Could you check a few things on this model? Use its own coordinates, in mm. A direction names the side the tool comes from. Give positions to 0.01 mm unless a question says otherwise; leave off trailing zeros. Loops run counter-clockwise (first coordinate to the right, second up) from the corner with the lowest first, then second, coordinate; pieces in that order, holes last. Notation, with made-up numbers: (56, -7.75) - (89, -7.75) arc R31 ccw to (89, 24.25) - close; hole circle Ø4 at (31, 22). An arc over 180 degrees is marked (long way). Use CSV: the item, a comma, the result in double quotes.
from build123d import *

# Parameters (mm, degrees)
SKETCH1_W           = 144
SKETCH1_H           = 125.68
BOSS_EXTRUDE1_DEPTH = 3
SKETCH2_W           = 144
SKETCH2_H           = 125.68
SKETCH2_W_2         = 140.282516161
SKETCH2_H_2         = 121.548177757
BOSS_EXTRUDE2_DEPTH = 83
SKETCH4_W           = 103.746737409
SKETCH4_H           = 37.953937335
CUT_EXTRUDE1_DEPTH  = 20
SKETCH5_W           = 110.713821745
SKETCH5_H           = 19.414835186
SKETCH5_H_2         = 24.021424071
CUT_EXTRUDE2_DEPTH  = 20
SKETCH6_W           = 39.790164022
SKETCH6_H           = 75.651590962
CUT_EXTRUDE3_DEPTH  = 20


with BuildPart() as part:
    # Sketch1 → Boss-Extrude1 (new body)
    with BuildSketch(Plane(origin=(0, 0, 0), x_dir=(1, 0, 0), z_dir=(0, 1, 0))):
        with Locations((-0.900426333, 18.508659662)):
            Rectangle(SKETCH1_W, SKETCH1_H)
    extrude(amount=BOSS_EXTRUDE1_DEPTH)

    # Sketch2 → Boss-Extrude2 (add)
    with BuildSketch(Plane(origin=(0, 3, 0), x_dir=(1, 0, 0), z_dir=(0, 1, 0))):
        with Locations((-0.900426333, 18.508659662)):
            Rectangle(SKETCH2_W, SKETCH2_H)
        with Locations((-1.012042147, 18.478566742)):
            Rectangle(SKETCH2_W_2, SKETCH2_H_2, mode=Mode.SUBTRACT)
    extrude(amount=BOSS_EXTRUDE2_DEPTH)

    # Sketch4 → Cut-Extrude1 (cut)
    with BuildSketch(Plane(origin=(71.099573667, 0, 0), x_dir=(0, 0, -1), z_dir=(1, 0, 0))):
        with Locations((16.534795252, 50.079604952)):
            Rectangle(SKETCH4_W, SKETCH4_H)
    extrude(amount=-CUT_EXTRUDE1_DEPTH, mode=Mode.SUBTRACT)

    # Sketch5 → Cut-Extrude2 (cut)
    with BuildSketch(Plane.XZ):
        with Locations((-5.028686967, -50.405830616)):
            Rectangle(SKETCH5_W, SKETCH5_H)
        with Locations((-5.028686967, 8.182044553)):
            Rectangle(SKETCH5_W, SKETCH5_H_2)
    extrude(amount=-CUT_EXTRUDE2_DEPTH, mode=Mode.SUBTRACT)

    # Sketch6 → Cut-Extrude3 (cut)
    with BuildSketch(Plane.ZY.offset(72.900426333)):
        with Locations((19.353212204, 44.793227562)):
            Rectangle(SKETCH6_W, SKETCH6_H)
    extrude(amount=-CUT_EXTRUDE3_DEPTH, mode=Mode.SUBTRACT)


solid = part.part
1) I need wall thicknesses on line 1 along Z through (x, y) = (-19, 12); line 2 along X through (y, z) = (8, -58); line 3 along Y through (x, z) = (38, 21.5). Which ranges of each line are inside material? Lowest first, please.
Answer below:
line 1,"z = -81.35 to -79.25, 42.3 to 44.33"
line 2,"x = -72.9 to -71.15, 69.13 to 71.1"
line 3,"y = 0 to 3"
2) Which directions (+Z, -Z, +X, -X, +Y, -Y) give clear straight access to the entire face, cutting with the end or side of a thin tool? Please do faces 1 (the flat face through (-72.9, 42, -32)), 2 (the flat face through (-2, 44, 42.296)).
Answer below:
face 1,"+Z, -Z, -X, +Y, -Y"
face 2,"+Y"
3) Suppose I cut it at D-D (x = 12). Please give me the cut outline in (y, z).
Answer below:
outline,"(0, -81.35) - (86, -81.35) - (86, -79.25) - (3, -79.25) - (3, -60.11) - (0, -60.11) - close; (0, -40.7) - (3, -40.7) - (3, -3.83) - (0, -3.83) - close; (0, 20.19) - (3, 20.19) - (3, 42.3) - (86, 42.3) - (86, 44.33) - (0, 44.33) - close"
4) I'm going to push a flat-ended pin straight in: P1, Ø10, axis at x = 44, z = -34, coming from the +Y side. Where does the tip first touch, or does it pass through?
Answer below:
P1,"stops at y = 3"
5) Suppose I cut it at A-A (z = 32). Please give me the cut outline in (x, y), plus the area to 3 significant figures.
Answer below:
outline,"(-72.9, 0) - (71.1, 0) - (71.1, 31.1) - (69.13, 31.1) - (69.13, 3) - (-71.15, 3) - (-71.15, 6.97) - (-72.9, 6.97) - close; (-72.9, 82.62) - (-71.15, 82.62) - (-71.15, 86) - (-72.9, 86) - close; (69.13, 69.06) - (71.1, 69.06) - (71.1, 86) - (69.13, 86) - close"
area,"534 mm2"
6) We'd pull the mould along Z, two halves only. Please class faces 3 (the flat face through (-2, 42, -81.349)), 4 (the flat face through (-2, 42, 44.331)), 5 (the flat face through (-2, 0, -19)), 6 (the flat face through (-2, 44, -79.253)): +Z half, -Z half, draft (parallel to the pull), parting line (faces both ways), or undercut.
Answer below:
face 3,"-Z half"
face 4,"+Z half"
face 5,"draft"
face 6,"undercut"
7) Suppose I cut it at C-C (z = 16). Please give me the cut outline in (x, y), plus the area to 3 significant figures.
Answer below:
outline,"(-72.9, 0) - (-60.39, 0) - (-60.39, 3) - (-71.15, 3) - (-71.15, 6.97) - (-72.9, 6.97) - close; (-72.9, 82.62) - (-71.15, 82.62) - (-71.15, 86) - (-72.9, 86) - close; (50.33, 0) - (71.1, 0) - (71.1, 31.1) - (69.13, 31.1) - (69.13, 3) - (50.33, 3) - close; (69.13, 69.06) - (71.1, 69.06) - (71.1, 86) - (69.13, 86) - close"
area,"201 mm2"
8) Suppose I cut it at B-B (y = 60.5). Please give me the cut outline in (x, z).
Answer below:
outline,"(-72.9, -81.35) - (71.1, -81.35) - (71.1, -68.41) - (69.13, -68.41) - (69.13, -79.25) - (-71.15, -79.25) - (-71.15, -0.54) - (-72.9, -0.54) - close; (-72.9, 39.25) - (-71.15, 39.25) - (-71.15, 42.3) - (69.13, 42.3) - (69.13, 35.34) - (71.1, 35.34) - (71.1, 44.33) - (-72.9, 44.33) - close"
